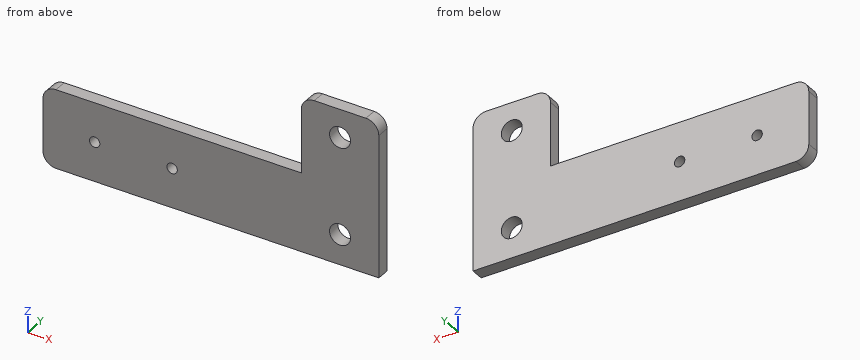
```python
from build123d import *

# Parameters (mm, degrees)
BOSS_EXTRUDE1_DEPTH = 6.35
CUT_EXTRUDE1_REACH  = 8.35
SKETCH4_R           = 2.5527
SKETCH4_R_2         = 5.1562
FILLET1_R           = 6.35


with BuildPart() as part:
    # Sketch3 → Boss-Extrude1 (new body)
    with BuildSketch(Plane(origin=(0, 0, 0), x_dir=(1, 0, 0), z_dir=(0, 1, 0))):
        Polygon((0, 0), (165.1, 0), (165.1, -76.2), (127, -76.2), (127, -38.608), (0, -38.608), align=None)
    extrude(amount=BOSS_EXTRUDE1_DEPTH)

    # Sketch4 → Cut-Extrude1 (cut, up to next)
    with BuildSketch(Plane(origin=(0, 6.35, 0), x_dir=(1, 0, 0), z_dir=(0, 1, 0)), mode=Mode.PRIVATE) as cut_extrude1_sk1:
        with Locations((25.4, -19.304)):
            Circle(SKETCH4_R)
    cut_extrude1_tool1 = extrude(cut_extrude1_sk1.sketch, amount=-CUT_EXTRUDE1_REACH, mode=Mode.PRIVATE) & part.part
    add(cut_extrude1_tool1.solids().sort_by_distance((25.4, 6.35, 19.304))[0], mode=Mode.SUBTRACT)
    # Sketch4 → Cut-Extrude1 (cut, up to next)
    with BuildSketch(Plane(origin=(0, 6.35, 0), x_dir=(1, 0, 0), z_dir=(0, 1, 0)), mode=Mode.PRIVATE) as cut_extrude1_sk2:
        with Locations((63.5, -19.304)):
            Circle(SKETCH4_R)
    cut_extrude1_tool2 = extrude(cut_extrude1_sk2.sketch, amount=-CUT_EXTRUDE1_REACH, mode=Mode.PRIVATE) & part.part
    add(cut_extrude1_tool2.solids().sort_by_distance((63.5, 6.35, 19.304))[0], mode=Mode.SUBTRACT)
    # Sketch4 → Cut-Extrude1 (cut, up to next)
    with BuildSketch(Plane(origin=(0, 6.35, 0), x_dir=(1, 0, 0), z_dir=(0, 1, 0)), mode=Mode.PRIVATE) as cut_extrude1_sk3:
        with Locations((146.05, -14.7955)):
            Circle(SKETCH4_R_2)
    cut_extrude1_tool3 = extrude(cut_extrude1_sk3.sketch, amount=-CUT_EXTRUDE1_REACH, mode=Mode.PRIVATE) & part.part
    add(cut_extrude1_tool3.solids().sort_by_distance((146.05, 6.35, 14.7955))[0], mode=Mode.SUBTRACT)
    # Sketch4 → Cut-Extrude1 (cut, up to next)
    with BuildSketch(Plane(origin=(0, 6.35, 0), x_dir=(1, 0, 0), z_dir=(0, 1, 0)), mode=Mode.PRIVATE) as cut_extrude1_sk4:
        with Locations((146.05, -62.4205)):
            Circle(SKETCH4_R_2)
    cut_extrude1_tool4 = extrude(cut_extrude1_sk4.sketch, amount=-CUT_EXTRUDE1_REACH, mode=Mode.PRIVATE) & part.part
    add(cut_extrude1_tool4.solids().sort_by_distance((146.05, 6.35, 62.4205))[0], mode=Mode.SUBTRACT)

    # Fillet1
    fillet1_edges = [part.edges().sort_by_distance(p)[0] for p in [
        (0, 3.175, 0),
        (165.1, 3.175, 76.2),
        (127, 3.175, 76.2),
        (0, 3.175, 38.608),
    ]]
    fillet(fillet1_edges, radius=FILLET1_R)


solid = part.part
```
Model file for the job. Use its own axes, mm. Coordinates: 2 decimals unless noted, no trailing zeros. Order: outer loops, then holes, each group sorted by start corner. A loop starts at its lowest first (then second) coordinate and runs counter-clockwise, first axis right, second up. Notation, with made-up numbers: (19, 56.25) -> (23, 56.25) arc R23 cw to (23, 71.25) -> close; hole circle Ø4 at (89.5, 57). An arc over 180 degrees is marked (long way). Answer as a JSON object with one key per item and string values. Group by question number.
1) Cut at D-D, the plane y = 5. Write the cut outline in (x, z).
2) Cut at C-C, the plane z = 64. Write the cut outline in (x, y).
3) Drill centre lines: L1, parallel to Z at x = 146.05, y = 4.75; L2, parallel to Z at x = 25.4, y = 3.75; L3, parallel to X at y = 4.75, z = 54. Where is each one in solid material? Low to high.
4) Cut at A-A, the plane x = 25.4. Write the cut outline in (y, z).
5) Cut at B-B, the plane x = 146.05. Write the cut outline in (y, z), then the cut area to 3 significant figures.
6) Flat gauge pins, fed straight in: pin 1 (8 mm diameter, centred on x = 146.05, z = 14.8, fed in from -Y); pin 2 (1.5 mm diameter, centred on x = 24, z = 37.5, fed in from -Y); pin 3 (1.9 mm diameter, centred on x = 49.5, y = 4, fed in from +Z). Where does each tip first touch, or does it go through?
Check values:
{
 "1": {"outline": "(0, 6.35) arc R6.35 ccw to (6.35, 0) -> (165.1, 0) -> (165.1, 69.85) arc R6.35 ccw to (158.75, 76.2) -> (133.35, 76.2) arc R6.35 ccw to (127, 69.85) -> (127, 38.61) -> (6.35, 38.61) arc R6.35 ccw to (0, 32.26) -> close; hole circle Ø5.11 at (25.4, 19.3); hole circle Ø5.11 at (63.5, 19.3); hole circle Ø10.31 at (146.05, 14.8); hole circle Ø10.31 at (146.05, 62.42)"},
 "2": {"outline": "(127, 0) -> (141.14, 0) -> (141.14, 6.35) -> (127, 6.35) -> close; (150.96, 0) -> (165.1, 0) -> (165.1, 6.35) -> (150.96, 6.35) -> close"},
 "3": {"L1": "z = 0 to 9.64, 19.95 to 57.26, 67.58 to 76.2", "L2": "z = 0 to 16.75, 21.86 to 38.61", "L3": "x = 127 to 165.1"},
 "4": {"outline": "(0, 0) -> (6.35, 0) -> (6.35, 16.75) -> (0, 16.75) -> close; (0, 21.86) -> (6.35, 21.86) -> (6.35, 38.61) -> (0, 38.61) -> close"},
 "5": {"outline": "(0, 0) -> (6.35, 0) -> (6.35, 9.64) -> (0, 9.64) -> close; (0, 19.95) -> (6.35, 19.95) -> (6.35, 57.26) -> (0, 57.26) -> close; (0, 67.58) -> (6.35, 67.58) -> (6.35, 76.2) -> (0, 76.2) -> close", "area": "353 mm²"},
 "6": {"pin 1": "passes through", "pin 2": "stops at y = 0", "pin 3": "stops at z = 38.61"}
}
